Can you work these out from the drawing? Everything is in mm from the part's minimum corner. Give positions to 0.01 mm unless a question says otherwise; leave off trailing zeros. Write each loop counter-clockwise with the first axis right and the second up, starting at its lowest first coordinate (ties: lowest second). Pieces come first, ordered by that corner, then holes. Notation, with made-up numbers: (61, 57) -> (70, 57) arc R25 cw to (70, 75) -> close; hole circle Ø3 at (-0.5, 0.25). An arc over 180 degrees is marked (long way). Use one line per item in the form item = value.
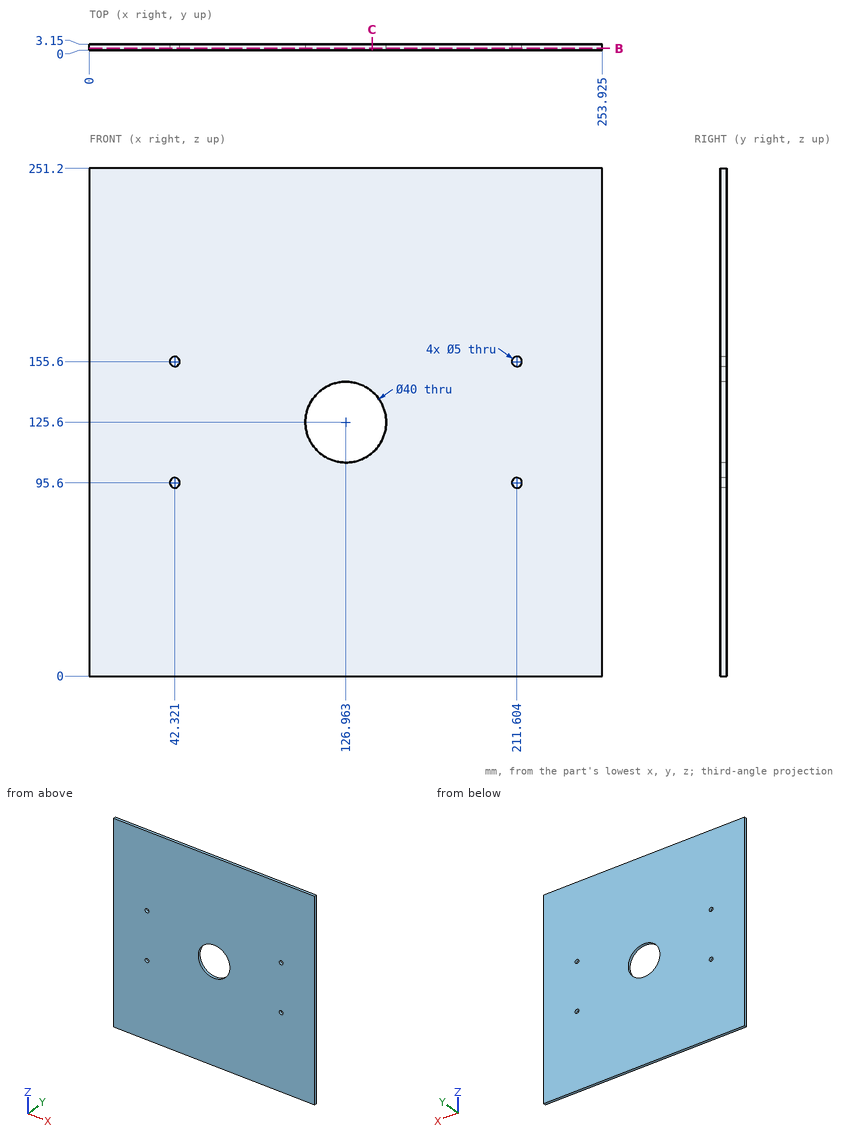
Q1. Will this pin go through, and if not, where does the flat tip stop? pin 1 Ø24 at (x, z) = (126.96, 125.6) entering from -Y.
Result set:
pin_1 = through
Q2. I want a section at C-C, the plane x = 140. Write out the boundary of the cut face in (y, z).
Result set:
outline = (0, 0) -> (3.15, 0) -> (3.15, 110.43) -> (0, 110.43) -> close; (0, 140.77) -> (3.15, 140.77) -> (3.15, 251.2) -> (0, 251.2) -> close
Q3. I want a section at B-B, the plane y = 0.95. Write out the boundary of the cut face in (x, z) (1 decimal).
Result set:
outline = (0, 0) -> (253.9, 0) -> (253.9, 251.2) -> (0, 251.2) -> close; hole circle Ø5 at (42.3, 95.6); hole circle Ø5 at (42.3, 155.6); hole circle Ø40 at (127, 125.6); hole circle Ø5 at (211.6, 95.6); hole circle Ø5 at (211.6, 155.6)
Q4. If I drill on line 1 along X through (y, z) = (1.35, 155.6) (1 decimal); line 2 along Z through (x, y) = (42.5, 0.75); line 3 along X through (y, z) = (0.8, 94) (1 decimal), over which ranges is the centre line in solid material (lowest first)? Write a range as from..to.
Result set:
line_1 = 0..39.8, 44.8..209.1, 214.1..253.9
line_2 = 0..93.11, 98.09..153.11, 158.09..251.2
line_3 = 0..40.4, 44.2..209.7, 213.5..253.9
